Work out the finished part from the listing and answer in its coordinate system (mm). Face numbers are marked on the shaded views. A direction names the side the tool comes from. Coordinates: 2 decimals unless noted, no trailing zeros. Write each loop counter-clockwise with the first axis right and the second up, starting at its lowest first coordinate (ties: lowest second). Pieces come first, ordered by that corner, then holes. Notation, with made-up numbers: M 59,35.25 L 73,35.25 A13 cw 73,47.25 Z; hole C 24,-29.75 d7. An arc over 180 degrees is marked long. Answer as CSV lines item,"result". Start each with the question number.
(1) Find the intervals of material crossed by L1, parallel to X at y = -60, z = -25; L2, parallel to Y at x = -30, z = -27.5, in increasing order. Write a range as [from, to].
(2) For the marked faces 5 and 6, determine the directions among +Z, -Z, +X, -X, +Y, -Y from which every point of the face is accessible in a straight line to the end or side of a thin tool.
(3) A cutting plane is placed at C-C on x = -16. Give the vertices of the cut face in (y, z).
(4) A cutting plane is placed at A-A on y = -62.5. Give the vertices of the cut face in (x, z), then the cut area to 3 significant figures.
(5) Flat-ended cylindrical pins translate along their axes: P1, Ø3, axis at x = -4.5, z = -39.5, coming from the +Y side; P2, Ø6.5, axis at x = -21, z = -37, coming from the -Y side. Find the tip coordinate at first contact, or state that the pin passes through.
(6) The mould has two halves that part along X. Classify the marked faces 1, 2, 3 and 4: released by +X, released by -X, zero draft, split by the parting line, or undercut.
(7) A cutting plane is placed at B-B on z = -20. Give the vertices of the cut face in (x, y), then the cut area to 3 significant figures.
from build123d import *

# Parameters (mm, degrees)
F0_W     = 40.843203
F0_H     = 38.1
F0_W_2   = 25.603201
F0_W_3   = 40.843199
F1_DEPTH = 76.2
F2_W     = 21.640803
F2_H     = 38.1
F3_DEPTH = 25.4


with BuildPart() as f1:
    # F0 (on Front) → F1 (new body)
    with BuildSketch(Plane.XZ):
        with Locations((-56.083202, -36.576001)):
            Rectangle(F0_W, F0_H)
        with Locations((-22.86, -36.576001)):
            Rectangle(F0_W_2, F0_H)
        with Locations((10.3632, -36.576001)):
            Rectangle(F0_W_3, F0_H)
    extrude(amount=F1_DEPTH)

    # F2 (on face) → F3 (cut)
    with BuildSketch(Plane.XZ.offset(76.2)):
        with Locations((-23.9268, -36.576001)):
            Rectangle(F2_W, F2_H)
    extrude(amount=-F3_DEPTH, mode=Mode.SUBTRACT)


solid = f1.part
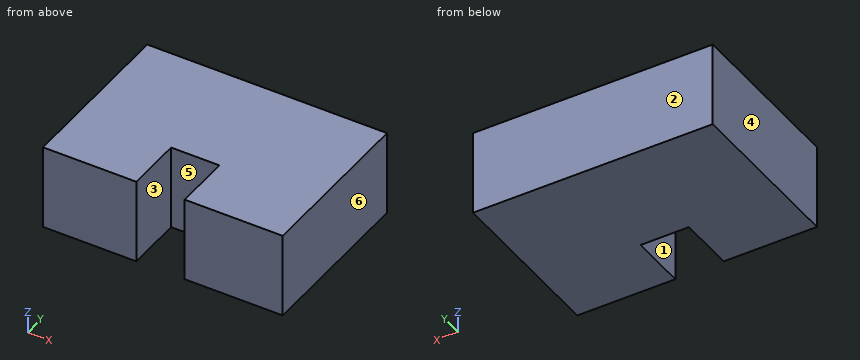
Here are the results:
1,L1,"x = [-76.5, -34.75], [-13.11, 30.78]"
1,L2,"y = [-50.8, 0]"
2,face 5,"+Z, -Z, -Y"
2,face 6,"+Z, -Z, +X, +Y, -Y"
3,outline,"M -50.8,-55.63 L 0,-55.63 L 0,-17.53 L -50.8,-17.53 Z"
4,outline,"M -76.5,-55.63 L -34.75,-55.63 L -34.75,-17.53 L -76.5,-17.53 Z; M -13.11,-55.63 L 30.78,-55.63 L 30.78,-17.53 L -13.11,-17.53 Z"
4,area,"3,260 mm^2"
5,P1,"stops at y = 0"
5,P2,"stops at y = -50.8"
6,face 1,"undercut"
6,face 2,"zero draft"
6,face 3,"undercut"
6,face 4,"released by -X"
7,outline,"M -76.5,-76.2 L -34.75,-76.2 L -34.75,-50.8 L -13.11,-50.8 L -13.11,-76.2 L 30.78,-76.2 L 30.78,0 L -76.5,0 Z"
7,area,"7,630 mm^2"
